Read the model definition and answer for the solid it produces. Units are mm, in the model's axes. A direction names the side the tool comes from. Round coordinates to 2 decimals unless told otherwise and drop trailing zeros. Order: outer loops, then holes, each group sorted by start corner. A loop starts at its lowest first (then second) coordinate and runs counter-clockwise, first axis right, second up. Notation, with made-up numbers: (18.25, -28.5) -> (71.25, -28.5) arc R20 ccw to (71.25, -8.5) -> close; hole circle Ø7 at (63.25, -15.5). An arc over 180 degrees is marked (long way). Use a Markdown table: item, result. Add a question column.
1. Section C-C, the plane x = 2.5 is taken. Give the vertices of the cut face in (y, z), then the cut area to 3 significant figures.
2. Consider L1, parallel to Z at x = 0, y = -2.25; L2, parallel to X at y = -7.5, z = 0; L3, parallel to Z at x = 3, y = -5.25. Determine where each line is inside the solid, lowest interval first. Write a range as [from, to].
3. Given pin 1 (1.5 mm diameter, centred on x = 4.5, y = -8, fed in from +Z); pin 2 (6 mm diameter, centred on x = -4.5, y = -5, fed in from -Z); pin 3 (2.5 mm diameter, centred on x = 2.5, y = -7, fed in from -Z); pin 4 (3 mm diameter, centred on y = -7, z = -8.5, fed in from +X), each flat-ended and moving along its own axis, determine where each tip first touches the part or whether it passes through.
4. Section D-D, the plane y = -8.5 is taken. Give the vertices of the cut face in (x, z).
5. For faces 1 (the face through (3.5, -2, -12)), 2 (the face through (4, -7, 7.9)), 3 (the face through (0.176, -2.465, 20.498)), 4 (the face through (4, -7, -7.9)), 5 (the face through (-0.176, -2.465, -20.498)), determine the directions among +Z, -Z, +X, -X, +Y, -Y from which every point of the face is accessible in a straight line to the end or side of a thin tool.
6. The mould has two halves that part along Y. Classify faces 6 (the face through (-3.5, -2, -13)), 7 (the face through (6.5, -6.6, -1.2)), 8 (the face through (-7, -5, -4)): +Y half, -Y half, draft (parallel to the pull), parting line (faces both ways), or undercut.
7. Section B-B, the plane y = -2 is taken. Give the vertices of the cut face in (x, z).
8. Section A-A, the plane z = 11.5 is taken. Give the vertices of the cut face in (x, y).
```python
from build123d import *

# Parameters (mm, degrees)
F1_DEPTH = 5
F3_DEPTH = 5
F4_R     = 2
F5_DEPTH = 6.1


with BuildPart() as f1:
    # F0 (on Front) → F1 (new body)
    with BuildSketch(Plane.XZ):
        with BuildLine():
            ThreePointArc((-8, -12.5), (0, -20.5), (8, -12.5))
            Line((8, -12.5), (8, 12.5))
            ThreePointArc((8, 12.5), (0, 20.5), (-8, 12.5))
            Line((-8, 12.5), (-8, -12.5))
        make_face()
        Polygon((0, -8.458548), (3.5, -10.479274), (3.5, -14.520726), (0, -16.541452), (-3.5, -14.520726), (-3.5, -10.479274), align=None, mode=Mode.SUBTRACT)
        with BuildLine():
            ThreePointArc((1.9, -1.774824), (-2.6, 0), (1.9, 1.774824))
            Line((1.9, 1.774824), (1.9, 3.5))
            Line((1.9, 3.5), (5, 3.5))
            Line((5, 3.5), (5, -3.5))
            Line((5, -3.5), (1.9, -3.5))
            Line((1.9, -3.5), (1.9, -1.774824))
        make_face(mode=Mode.SUBTRACT)
        Polygon((0, 16.541452), (3.5, 14.520726), (3.5, 10.479274), (0, 8.458548), (-3.5, 10.479274), (-3.5, 14.520726), align=None, mode=Mode.SUBTRACT)
    extrude(amount=F1_DEPTH)

    # F2 (on face) → F3 (join)
    with BuildSketch(Plane.XZ.offset(5)):
        with BuildLine():
            Line((8, 7.9), (0, 7.9))
            ThreePointArc((0, 7.9), (-7.9, 0), (0, -7.9))
            Line((0, -7.9), (8, -7.9))
            Line((8, -7.9), (8, 7.9))
        make_face()
        with BuildLine():
            ThreePointArc((1.9, -1.774824), (-2.6, 0), (1.9, 1.774824))
            Line((1.9, 1.774824), (1.9, 3.5))
            Line((1.9, 3.5), (5, 3.5))
            Line((5, 3.5), (5, -3.5))
            Line((5, -3.5), (1.9, -3.5))
            Line((1.9, -3.5), (1.9, -1.774824))
        make_face(mode=Mode.SUBTRACT)
    extrude(amount=F3_DEPTH)

    # F4 (on face) → F5 (cut, through all)
    with BuildSketch(Plane.YZ.offset(8)):
        with Locations((-5, 0)):
            Circle(F4_R)
    extrude(amount=-F5_DEPTH, mode=Mode.SUBTRACT)


solid = f1.part
```
Verdict:
| question | item | result |
|---|---|---|
| 1 | outline | (-10, -7.9) -> (-5, -7.9) -> (-5, -9.9) -> (0, -9.9) -> (0, -3.5) -> (-10, -3.5) -> close; (-10, 3.5) -> (0, 3.5) -> (0, 9.9) -> (-5, 9.9) -> (-5, 7.9) -> (-10, 7.9) -> close; (-5, -20.1) -> (0, -20.1) -> (0, -15.1) -> (-5, -15.1) -> close; (-5, 15.1) -> (0, 15.1) -> (0, 20.1) -> (-5, 20.1) -> close |
| 1 | area | 158 mm2 |
| 2 | L1 | z = [-20.5, -16.54], [-8.46, -2.6], [2.6, 8.46], [16.54, 20.5] |
| 2 | L2 | x = [-7.9, -2.6], [5, 8] |
| 2 | L3 | z = [-7.9, -3.5], [3.5, 7.9] |
| 3 | pin 1 | stops at z = 7.9 |
| 3 | pin 2 | stops at z = -20.36 |
| 3 | pin 3 | stops at z = -7.9 |
| 3 | pin 4 | stops at x = 8 |
| 4 | outline | (0, -7.9) -> (8, -7.9) -> (8, 7.9) -> (0, 7.9) arc R7.9 ccw to start; hole (1.9, -3.5) -> (5, -3.5) -> (5, 3.5) -> (1.9, 3.5) -> (1.9, 1.77) arc R2.6 ccw (long way) to (1.9, -1.77) -> close |
| 5 | face 1 | +Y, -Y |
| 5 | face 2 | +Z, +X, -X, -Y |
| 5 | face 3 | +Z, +Y, -Y |
| 5 | face 4 | -Z, +X, -X, -Y |
| 5 | face 5 | -Z, +Y, -Y |
| 6 | face 6 | draft |
| 6 | face 7 | undercut |
| 6 | face 8 | -Y half |
| 7 | outline | (-8, -12.5) arc R8 ccw to (8, -12.5) -> (8, 12.5) arc R8 ccw to (-8, 12.5) -> close; hole (-3.5, -14.52) -> (0, -16.54) -> (3.5, -14.52) -> (3.5, -10.48) -> (0, -8.46) -> (-3.5, -10.48) -> close; hole (-3.5, 10.48) -> (0, 8.46) -> (3.5, 10.48) -> (3.5, 14.52) -> (0, 16.54) -> (-3.5, 14.52) -> close; hole (1.9, -3.5) -> (5, -3.5) -> (5, 3.5) -> (1.9, 3.5) -> (1.9, 1.77) arc R2.6 ccw (long way) to (1.9, -1.77) -> close |
| 8 | outline | (-8, -5) -> (-3.5, -5) -> (-3.5, 0) -> (-8, 0) -> close; (3.5, -5) -> (8, -5) -> (8, 0) -> (3.5, 0) -> close |
